Read the model definition and answer for the solid it produces. Units are mm, in the model's axes. A direction names the side the tool comes from. Coordinates: 2 decimals unless noted, no trailing zeros. Write each loop counter-clockwise with the first axis right and the second up, starting at its lowest first coordinate (ties: lowest second). Pieces come first, ordered by that corner, then holes. Notation, with made-up numbers: (-22, 55.25) -> (-7, 55.25) arc R24 cw to (-7, 68.25) -> close; hole circle Ø9 at (79.25, 32). An arc over 180 degrees is marked (long way). Return JSON: item names as keys, results as strings.
Autodesk Inventor part; units mm, degrees
ref_plane "YZ Plane" through (0, 0, 0) normal (1, 0, 0) x (0, 1, 0)
ref_plane "XZ Plane" through (0, 0, 0) normal (0, 1, 0) x (-1, 0, 0)
ref_plane "XY Plane" through (0, 0, 0) normal (0, 0, 1) x (1, 0, 0)
sketch "Sketch1" plane through (0, 0, 0) normal (0, 1, 0) x (-1, 0, 0)
  line L0 (90, 0) -> (90, -90)
  line L1 (0, -90) -> (0, 0)
  line L2 (90, 0) -> (90, -90)
  line L3 (90, -90) -> (0, -90)
  line L4 (10, -180) -> (80, -180)
  line L5 (90, 0) -> (80, 0)
  line L6 (80, 0) -> (80, -90)
  line L7 (0, 0) -> (10, 0)
  line L8 (10, 0) -> (10, -90)
  line L9 (80, -270) -> (80, -180)
  line L10 (10, -270) -> (10, -180)
  line L11 (80, -270) -> (70, -270)
  line L12 (70, -270) -> (70, -180)
  line L13 (10, -270) -> (20, -270)
  line L14 (20, -270) -> (20, -180)
  line L15 (80, -90) -> (70, -90)
  line L16 (70, -180) -> (60, -180)
  line L17 (20, -180) -> (30, -180)
  line L18 (70, -180) -> (70, -90)
  line L19 (20, -180) -> (20, -90)
  line L20 (80, -270) -> (70, -270)
  line L21 (20, -270) -> (10, -270)
  line L22 (0, 0) -> (10, 0)
  line L23 (80, 0) -> (90, 0)
  line L24 (90, 0) -> (80, 0)
  line L25 (0, 0) -> (10, 0)
  line L26 (90, 0) -> (0, 0)
  line L27 (80, -270) -> (10, -270)
  dimension "d2" = 90
  dimension "d4" = 10
  dimension "d5" = 10
extrude "Extrusion1" add sketch "Sketch1" along normal blind 50
sketch "Sketch2" plane through (0, 50, 0) normal (0, 1, 0) x (1, 0, 0)
  arc A0 (-10, 59.3649) -> (-80, 59.3649) centre (-45, 40) ccw
  line L0 (-90, 0) -> (0, 0)
  line L1 (-90, 0) -> (-80, 0)
  line L2 (-80, 0) -> (-80, 59.3649)
  line L3 (0, 0) -> (-10, 0)
  line L4 (-10, 0) -> (-10, 59.3649)
  line L5 (-80, 0) -> (-10, 0)
  line L6 (-80, 270) -> (-80, 180)
  line L7 (-70, 270) -> (-20, 270)
  line L8 (-80, 180) -> (-80, 190)
  line L9 (-10, 180) -> (-10, 270)
  line L10 (-70, 270) -> (-70, 215)
  line L11 (-20, 270) -> (-20, 215)
  arc A1 (-70, 215) -> (-20, 215) centre (-45, 215) ccw
  point P0 (-90, 90)
  dimension "d18" = 10
  dimension "d19" = 10
  dimension "d25" = 10
extrude "Extrusion2" cut sketch "Sketch2" against normal blind 50
fillet "Fillet1" radius 10 1 edges at (-70, 25, -90)
fillet "Fillet2" radius 10 1 edges at (-90, 25, -90)
fillet "Fillet3" radius 10 2 edges at (-20, 25, -90) (0, 25, -90)
fillet "Fillet4" radius 5 1 edges at (-80, 25, -180)
fillet "Fillet5" radius 5 3 edges at (-70, 25, -180) (-10, 25, -180) (-20, 25, -180)
sketch "Sketch3" plane through (-90, 0, 0) normal (-1, 0, 0) x (0, 0, 1)
  line L0 (0, 0) -> (0, 50)
  circle A0 centre (-20, 25) radius 2.5
  arc A1 (-8.775, 0) -> (-8.775, 50) centre (-40, 25) ccw
  line L1 (-80, 0) -> (-90, 0)
  line L2 (-8.775, 0) -> (0, 0)
  line L3 (0, 0) -> (0, 50)
  line L4 (0, 50) -> (-8.775, 50)
  line L5 (-270, 0) -> (-270, 50)
  circle A2 centre (-250, 25) radius 2.5
  line L6 (-270, 50) -> (-270, 0)
  arc A3 (-261.225, 50) -> (-261.225, 0) centre (-230, 25) ccw
  line L7 (-270, 0) -> (-261.225, 0)
  line L8 (-185, 0) -> (-270, 0)
  line L9 (-270, 50) -> (-261.225, 50)
  line L10 (-270, 50) -> (-185, 50)
  point P0 (0, 25)
  point P1 (-270, 25)
  dimension "d36" = 5
  dimension "d40" = 5
extrude "Extrusion3" cut sketch "Sketch3" against normal blind 150.25
sketch "Sketch4" plane through (-20, 0, -215) normal (-1, 0, 0) x (0, 0, 1)
  circle A0 centre (-35, 25) radius 2.5
  line L0 (-45, 25) -> (-45, 32.5)
  line L1 (-45, 32.5) -> (-15, 32.5)
  line L2 (-15, 32.5) -> (-15, 17.5)
  line L3 (-15, 17.5) -> (-45, 17.5)
  line L4 (-45, 25) -> (-45, 17.5)
  point P0 (215, 0)
  dimension "d43" = 10
  dimension "d44" = 7.5
  dimension "d45" = 30
  dimension "d47" = 15
extrude "Extrusion4" cut sketch "Sketch4" against normal blind 5
sketch "Sketch5" plane through (-20, 0, -215) normal (-1, 0, 0) x (0, 0, 1)
  line L0 (-45, 17.5) -> (-45, 32.5)
  line L1 (-45, 32.5) -> (-45, 35)
  line L2 (-15, 17.5) -> (-45, 17.5)
  line L3 (-45, 17.5) -> (-45, 15)
  line L4 (-45, 15) -> (-5, 15)
  line L5 (-5, 15) -> (-5, 35)
  line L6 (-5, 35) -> (-45, 35)
  line L7 (-45, 17.5) -> (-45, 32.5)
  point P0 (215, 0)
  dimension "d50" = 2.5
  dimension "d51" = 2.5
  dimension "d52" = 40
  dimension "d53" = 20
extrude "Extrusion5" cut sketch "Sketch5" against normal blind 5
properties part number "PartArmNEW"
1. A tool of negligible diameter and unlimited length cuts with its end or side. For faces 4 (the face through (-18, 15, -240)), 5 (the face through (-80, 25, -29)), 6 (the face through (-12, 25, -181)), 7 (the face through (-70, 25, -243)), from which of +Z, -Z, +X, -X, +Y, -Y can it reach the whole face along a straight path? Write none if from no direction.
Taken from the geometry:
{"face 4": "none", "face 5": "+Z, +Y, -Y", "face 6": "+X, +Y, -Y", "face 7": "-Z, +Y, -Y"}
2. Consider L1, parallel to Y at x = -84, z = -20; L2, parallel to X at y = 14, z = -41; L3, parallel to X at y = 6.5, z = -222.5. Determine where each line is inside the solid, lowest interval first.
Taken from the geometry:
{"L1": "y = 0 to 22.5, 27.5 to 50", "L2": "x = -90 to -80, -10 to 0", "L3": "x = -80 to -70, -20 to -10"}
3. The part is cut by section B-B (y = 25). Count the separate pieces of the cut face and the enclosed holes in it, then the cut area to 3 significant figures.
Taken from the geometry:
{"separate pieces": "5", "enclosed holes": "0", "area": "9,610 mm2"}
4. The part is cut by section D-D (x = -45). Determine the outline of the cut face in (y, z).
Taken from the geometry:
{"outline": "(0, -190) -> (50, -190) -> (50, -80) -> (0, -80) -> close"}
5. The part is cut by section A-A (z = -250). Determine the outline of the cut face in (x, y).
Taken from the geometry:
{"outline": "(-80, 0) -> (-70, 0) -> (-70, 22.5) -> (-80, 22.5) -> close; (-80, 27.5) -> (-70, 27.5) -> (-70, 50) -> (-80, 50) -> close; (-20, 0) -> (-10, 0) -> (-10, 22.5) -> (-15, 22.5) -> (-15, 15) -> (-20, 15) -> close; (-20, 35) -> (-15, 35) -> (-15, 27.5) -> (-10, 27.5) -> (-10, 50) -> (-20, 50) -> close"}
6. Flat-ended cylindrical pins translate along their axes: pin 1 Ø10 at (x, y) = (-40.5, 17.5) entering from -Z; pin 2 Ø16 at (y, z) = (22.5, -245.5) entering from -X; pin 3 Ø12 at (y, z) = (25, -147.5) entering from -X. Find the tip coordinate at first contact, or state that the pin passes through.
Taken from the geometry:
{"pin 1": "stops at z = -191.88", "pin 2": "stops at x = -80", "pin 3": "stops at x = -70"}
7. The part is cut by section C-C (z = -209). Determine the outline of the cut face in (x, y).
Taken from the geometry:
{"outline": "(-80, 0) -> (-69.27, 0) -> (-69.27, 50) -> (-80, 50) -> close; (-20.73, 0) -> (-10, 0) -> (-10, 50) -> (-20.73, 50) -> close"}
8. For a pull along Y with two mould halves and no side action, classify faces 1 (the face through (-18, 25, -260)), 2 (the face through (-15, 25, -270)), 3 (the face through (-79, 25, -182)) as +Y half, -Y half, draft (parallel to the pull), parting line (faces both ways), or undercut.
Taken from the geometry:
{"face 1": "undercut", "face 2": "parting line", "face 3": "draft"}
